For this review, take the finished solid that the model builds, in its own axes (mm). Coordinates: 2 decimals unless noted, no trailing zeros. Write each loop counter-clockwise with the first axis right and the second up, starting at its lowest first coordinate (ties: lowest second). Pieces come first, ordered by that corner, then holes.
```python
from build123d import *

# Parameters (mm, degrees)
F1_DEPTH = 836
F2_R     = 6.25
F3_DEPTH = 25.001


with BuildPart() as f1:
    # F0 (on Front) → F1 (new body, symmetric)
    with BuildSketch(Plane.XZ):
        with BuildLine():
            ThreePointArc((12.5, 7.5), (11.035534, 11.035534), (7.5, 12.5))
            Line((7.5, 12.5), (-7.5, 12.5))
            ThreePointArc((-7.5, 12.5), (-11.035534, 11.035534), (-12.5, 7.5))
            Line((-12.5, 7.5), (-12.5, -7.5))
            ThreePointArc((-12.5, -7.5), (-11.035534, -11.035534), (-7.5, -12.5))
            Line((-7.5, -12.5), (7.5, -12.5))
            ThreePointArc((7.5, -12.5), (11.035534, -11.035534), (12.5, -7.5))
            Line((12.5, -7.5), (12.5, 7.5))
        make_face()
        with BuildLine():
            Line((-7.5, 10), (7.5, 10))
            ThreePointArc((7.5, 10), (9.267767, 9.267767), (10, 7.5))
            Line((10, 7.5), (10, -7.5))
            ThreePointArc((10, -7.5), (9.267767, -9.267767), (7.5, -10))
            Line((7.5, -10), (-7.5, -10))
            ThreePointArc((-7.5, -10), (-9.267767, -9.267767), (-10, -7.5))
            Line((-10, -7.5), (-10, 7.5))
            ThreePointArc((-10, 7.5), (-9.267767, 9.267767), (-7.5, 10))
        make_face(mode=Mode.SUBTRACT)
    extrude(amount=F1_DEPTH, both=True)

    # F2 (on face) → F3 (cut, through all)
    with BuildSketch(Plane.YZ.offset(12.5)):
        with Locations((-816, 0)):
            Circle(F2_R)
        with Locations((816, 0)):
            Circle(F2_R)
    extrude(amount=-F3_DEPTH, mode=Mode.SUBTRACT)


solid = f1.part
```
Q1. Add section C-C (x = 3). State the section outline as (y, z) points.
Ans:
outline: (-836, -12.5) - (836, -12.5) - (836, -10) - (-836, -10) - close; (-836, 10) - (836, 10) - (836, 12.5) - (-836, 12.5) - close
Q2. Add section B-B (z = 0). State the section outline as (x, y) points, then the cut area to 4 significant figures.
Ans:
outline: (-12.5, -836) - (-10, -836) - (-10, -822.25) - (-12.5, -822.25) - close; (-12.5, -809.75) - (-10, -809.75) - (-10, 809.75) - (-12.5, 809.75) - close; (-12.5, 822.25) - (-10, 822.25) - (-10, 836) - (-12.5, 836) - close; (10, -836) - (12.5, -836) - (12.5, -822.25) - (10, -822.25) - close; (10, -809.75) - (12.5, -809.75) - (12.5, 809.75) - (10, 809.75) - close; (10, 822.25) - (12.5, 822.25) - (12.5, 836) - (10, 836) - close
area: 8,235 mm2
Q3. Clearance check with a flat-ended pin moving along its axis: pin 1 Ø11 at (y, z) = (-816, 0) entering from -X. State where the tip first meets the part, or that it passes through.
Ans:
pin 1: passes through
Q4. For probe 1 along Y at (x, z) = (-10.25, 1.25); probe 2 along X at (y, z) = (234, -3.5), list the stretches that pass through material, from the lowest coordinate up.
Ans:
probe 1: y = -836 to -822.12, -809.88 to 809.88, 822.12 to 836
probe 2: x = -12.5 to -10, 10 to 12.5
Q5. Add section A-A (y = -178.5). State the section outline as (x, z) points.
Ans:
outline: (-12.5, -7.5) arc R5 ccw to (-7.5, -12.5) - (7.5, -12.5) arc R5 ccw to (12.5, -7.5) - (12.5, 7.5) arc R5 ccw to (7.5, 12.5) - (-7.5, 12.5) arc R5 ccw to (-12.5, 7.5) - close; hole (-10, -7.5) arc R2.5 ccw to (-7.5, -10) - (7.5, -10) arc R2.5 ccw to (10, -7.5) - (10, 7.5) arc R2.5 ccw to (7.5, 10) - (-7.5, 10) arc R2.5 ccw to (-10, 7.5) - close
